from build123d import *

# Parameters (mm, degrees)
PAD001_DEPTH = 0.19
PAD_DEPTH    = 8
PAD002_DEPTH = 0.24


with BuildPart() as pad001:
    # Sketch001 → Pad001 (new body, symmetric)
    with BuildSketch(Plane.XZ):
        Polygon((0.25, -2.46), (-0.25, -2.46), (-0.25, 0.5), (1.02, 2.4), (1.02, 3.04), (1.52, 3.04), (1.52, 2.4), (0.25, 0.5), align=None)
        Polygon((3.56, 3.04), (4.06, 3.04), (4.06, 2.4), (5.37, 0.5), (5.37, -2.46), (4.87, -2.46), (4.87, 0.5), (3.56, 2.4), align=None)
    extrude(amount=PAD001_DEPTH, both=True)


with BuildPart() as pad:
    # Sketch → Pad (new body)
    with BuildSketch(Plane.XY.offset(3)):
        with BuildLine():
            Line((0.524231, -1.33), (4.555769, -1.33))
            ThreePointArc((4.555769, -1.33), (2.54, 2.415), (0.524231, -1.33))
        make_face()
    extrude(amount=PAD_DEPTH)


with BuildPart() as to_92_wide:
    # Sketch002 → Pad002 (new body, symmetric)
    with BuildSketch(Plane.YZ.offset(2.54)):
        Polygon((-0.19, 3), (0.19, 3), (0.19, 2.7), (2.73, 1.2), (2.73, -2.5), (2.35, -2.5), (2.35, 1), (-0.19, 2.5), align=None)
    extrude(amount=PAD002_DEPTH, both=True)

    add(pad001.part)
    add(pad.part)


solid = to_92_wide.part
Geometry: final body of the model. Coordinates: model frame, mm. A direction names the side the tool comes from. Give positions to 0.01 mm unless a question says otherwise; leave off trailing zeros. Write each loop counter-clockwise with the first axis right and the second up, starting at its lowest first coordinate (ties: lowest second). Pieces come first, ordered by that corner, then holes. Notation, with made-up numbers: (30.5, 88) - (62.5, 88) arc R21 ccw to (62.5, 124) - close; hole circle Ø11 at (-21.5, 9.25). An arc over 180 degrees is marked (long way). Return JSON: item names as keys, results as strings. Group by question number.
1) Section C-C on y = 2. Return the cut outline in (x, z).
2) First-contact query: P1, Ø1.4, axis at x = 0.5, z = 0, coming from the -Y side; P2, Ø1, axis at y = 0, z = 3.5, coming from the +X side (3 decimals); P3, Ø1.4, axis at x = 4.5, z = -0.5, coming from the +Y side. Flat tips, straight axial feed; report the tip coordinate or a pass-through.
3) Line query: line 1 (Z direction, x = 0.6, y = 0.85); line 2 (Z direction, x = 0.35, y = 0); line 3 (Y direction, x = 4.45, z = 3.5). Output: solid intervals per line, ascending.
4) Section B-B on x = 2.54. Return the cut outline in (y, z) (3 decimals).
5) Section D-D on x = 0.4. Return the cut outline in (y, z), plus the area to 3 significant figures.
6) Section A-A on z = -1. Return the cut outline in (x, y).
7) Set-up query: faces 5 (the flat face through (0.38, 0, 1.44)), 6 (the flat face through (4.71, 0, 1.46)), 7 (the flat face through (0, -0.19, 0)), 8 (the flat face through (2.54, 1.44, 1.96)). Return all of +Z, -Z, +X, -X, +Y, -Y with unobstructed straight access to the full face (end or side cutting, diameter ignored); none if empty.
8) Mould query, pull axis X, two halves, no side actions, for faces 1 (the cylindrical face through (2.613, 2.414, 6.944)), 2 (the flat face through (0.89, 0, 1.46)), 3 (the flat face through (0, 0.19, 0)), 4 (the flat face through (4.22, 0, 1.44)). Classes: released by +X, released by -X, zero draft, split by the parting line, or undercut.
Filled in:
{
 "1": {"outline": "(1.19, 3) - (3.89, 3) - (3.89, 11) - (1.19, 11) - close; (2.3, 1.21) - (2.78, 1.21) - (2.78, 1.63) - (2.3, 1.63) - close"},
 "2": {"P1": "stops at y = -0.19", "P2": "stops at x = 4.955", "P3": "stops at y = 0.19"},
 "3": {"line 1": "z = 3 to 11", "line 2": "z = 0.65 to 1.4, 3 to 11", "line 3": "y = -1.33 to 1.48"},
 "4": {"outline": "(-1.33, 3) - (-0.19, 3) - (-0.19, 2.5) - (2.35, 1) - (2.35, -2.5) - (2.73, -2.5) - (2.73, 1.2) - (0.19, 2.7) - (0.19, 3) - (2.415, 3) - (2.415, 11) - (-1.33, 11) - close"},
 "5": {"outline": "(-1.12, 3) - (1.12, 3) - (1.12, 11) - (-1.12, 11) - close; (-0.19, 0.72) - (0.19, 0.72) - (0.19, 1.47) - (-0.19, 1.47) - close", "area": "18.2 mm^2"},
 "6": {"outline": "(-0.25, -0.19) - (0.25, -0.19) - (0.25, 0.19) - (-0.25, 0.19) - close; (2.3, 2.35) - (2.78, 2.35) - (2.78, 2.73) - (2.3, 2.73) - close; (4.87, -0.19) - (5.37, -0.19) - (5.37, 0.19) - (4.87, 0.19) - close"},
 "7": {"face 5": "-X, +Y, -Y", "face 6": "+X, +Y, -Y", "face 7": "-Z, +X, -X, -Y", "face 8": "+X, -X, +Y"},
 "8": {"face 1": "split by the parting line", "face 2": "undercut", "face 3": "zero draft", "face 4": "undercut"}
}
